```python
from build123d import *

# Parameters (mm, degrees)
BOSS_EXTRUDE1_DEPTH = 3
BOSS_EXTRUDE2_DEPTH = 40


with BuildPart() as part:
    # Sketch1 → Boss-Extrude1 (new body)
    with BuildSketch(Plane(origin=(0, 0, 0), x_dir=(0, 0, -1), z_dir=(1, 0, 0))):
        Polygon((0, 74.865), (0, -74.865), (298, -65.13), (298, 65.13), align=None)
    extrude(amount=BOSS_EXTRUDE1_DEPTH)

    # Sketch2 → Boss-Extrude2 (add)
    with BuildSketch(Plane(origin=(3, 0, 0), x_dir=(0, 0, -1), z_dir=(1, 0, 0))):
        Polygon((0, 74.865), (298, 65.13), (298, 56.53), (298, 0), (289.4, 0), (289.4, 56.810942953), (252.6, 58.01311745), (252.6, 0), (244, 0), (244, 58.294060403), (54, 64.500939597), (54, 0), (45.4, 0), (45.4, 64.78188255), (8.6, 65.984057047), (8.6, 0), (0, 0), (0, 66.265), align=None)
    boss_extrude2 = extrude(amount=BOSS_EXTRUDE2_DEPTH)

    # Mirror1: Boss-Extrude2 across plane
    add(boss_extrude2.mirror(Plane(origin=(43, 0, -45.4), x_dir=(0, 0, 1), z_dir=(0, 1, 0))))


solid = part.part
```
For this review, take the finished solid that the model builds, in its own axes (mm). A direction names the side the tool comes from. Coordinates: 2 decimals unless noted, no trailing zeros. Order: outer loops, then holes, each group sorted by start corner. A loop starts at its lowest first (then second) coordinate and runs counter-clockwise, first axis right, second up. Notation, with made-up numbers: (29.25, 43) -> (78.25, 43) arc R35 cw to (78.25, 82) -> close; hole circle Ø8 at (74, 69.25). An arc over 180 degrees is marked (long way). Use CSV: the item, a comma, the result in double quotes. Start each with the question number.
Item 1: We need section C-C, the plane z = -22. Give the boundary of the cut face in (x, y).
Item 2: We need section D-D, the plane z = -206. Give the boundary of the cut face in (x, y), then the cut area to 3 significant figures.
Item 3: Insertion check: pin 1 (4 mm diameter, centred on x = 24, z = -213, fed in from -Y); pin 2 (11 mm diameter, centred on y = -13.5, z = -27, fed in from +X); pin 3 (1 mm diameter, centred on x = 37.5, z = -72.5, fed in from -Y). Each pin has a flat end and moves straight along its axis. Give the tip position at first contact, or say it passes through.
Item 4: Draft analysis for pull direction Y (two halves, no side actions). For faces 3 (the face through (3, 1, -271)), 4 (the face through (0, 1, -147)), 5 (the face through (3, 1, -27)), state which applies: pulls with the +Y half, pulls with the -Y half, needs draft (parallel to the pull), parting line crosses it, or undercut.
Item 5: We need section A-A, the plane x = 32. Give the boundary of the cut face in (y, z) (3 decimals).
Item 6: For faces 1 (the face through (23, 1, -289.4)), 2 (the face through (21, 1, -298)), list the 3-axis set-ups (+Z, -Z, +X, -X, +Y, -Y) from which the entire face can be reached by the end or side of a thin tool; tool diameter is ignored.
Item 7: We need section B-B, the plane y = -12.5. Give the boundary of the cut face in (x, z), then the cut area to 3 significant figures.
Item 8: Wall thickness on probe 1 along Z at (x, y) = (30.5, -22); probe 2 along X at (y, z) = (-9, -273.5); probe 3 along Y at (x, z) = (7.5, -15.5): over which ranges is each line inside the solid? List them lowest first.
Derived:
1,outline,"(0, -74.15) -> (43, -74.15) -> (43, -65.55) -> (3, -65.55) -> (3, 65.55) -> (43, 65.55) -> (43, 74.15) -> (0, 74.15) -> close"
2,outline,"(0, -68.14) -> (43, -68.14) -> (43, -59.54) -> (3, -59.54) -> (3, 59.54) -> (43, 59.54) -> (43, 68.14) -> (0, 68.14) -> close"
2,area,"1,100 mm^2"
3,pin 1,"stops at y = -67.97"
3,pin 2,"stops at x = 3"
3,pin 3,"stops at y = -72.51"
4,face 3,"undercut"
4,face 4,"needs draft"
4,face 5,"undercut"
5,outline,"(-74.865, 0) -> (-65.13, -298) -> (65.13, -298) -> (74.865, 0) -> close; hole (-65.984, -8.6) -> (-64.782, -45.4) -> (64.782, -45.4) -> (65.984, -8.6) -> close; hole (-64.501, -54) -> (-58.294, -244) -> (58.294, -244) -> (64.501, -54) -> close; hole (-58.013, -252.6) -> (-56.811, -289.4) -> (56.811, -289.4) -> (58.013, -252.6) -> close"
6,face 1,"+X"
6,face 2,"-Z, +X, -X, +Y, -Y"
7,outline,"(0, -298) -> (43, -298) -> (43, -289.4) -> (3, -289.4) -> (3, -252.6) -> (43, -252.6) -> (43, -244) -> (3, -244) -> (3, -54) -> (43, -54) -> (43, -45.4) -> (3, -45.4) -> (3, -8.6) -> (43, -8.6) -> (43, 0) -> (0, 0) -> close"
7,area,"2,270 mm^2"
8,probe 1,"z = -298 to -289.4, -252.6 to -244, -54 to -45.4, -8.6 to 0"
8,probe 2,"x = 0 to 3"
8,probe 3,"y = -74.36 to -65.76, 65.76 to 74.36"
